```python
from build123d import *

# Parameters (mm, degrees)
SKETCH1_W           = 24
SKETCH1_H           = 24
BOSS_EXTRUDE1_DEPTH = 20
SKETCH5_W           = 5
SKETCH5_H           = 4
SKETCH3_W           = 20
SKETCH3_H           = 20
CUT_EXTRUDE5_DEPTH  = 6
SKETCH14_W          = 20
SKETCH14_H          = 20
CUT_EXTRUDE6_DEPTH  = 2
CUT_EXTRUDE7_REACH  = 14
SKETCH15_W          = 17.5
SKETCH15_H          = 17.5


with BuildPart() as part:
    # Sketch1 → Boss-Extrude1 (new body)
    with BuildSketch(Plane(origin=(0, 0, 0), x_dir=(1, 0, 0), z_dir=(0, 1, 0))):
        Rectangle(SKETCH1_W, SKETCH1_H)
    extrude(amount=BOSS_EXTRUDE1_DEPTH)

    # Sweep1: sweep along a path in Sketch6
    with BuildLine(Plane(origin=(0, 0, 0), x_dir=(0, 0, -1), z_dir=(1, 0, 0))) as sweep1_path:
        Line((12, 16), (15, 16))
        ThreePointArc((15, 16), (17.025627927, 16.352272006), (18.813398517, 17.367722833))
    # Sketch5 → Sweep1 (sweep)
    with BuildSketch(Plane(origin=(0, 0, -12), x_dir=(-1, 0, 0), z_dir=(0, 0, -1))):
        with Locations((0, 16)):
            Rectangle(SKETCH5_W, SKETCH5_H)
    sweep1 = sweep(path=sweep1_path.line)

    # Mirror1: Sweep1 across plane
    add(sweep1.mirror(Plane.XY))

    # Sketch3 → Cut-Extrude5 (cut)
    with BuildSketch(Plane.XZ):
        Rectangle(SKETCH3_W, SKETCH3_H)
    extrude(amount=-CUT_EXTRUDE5_DEPTH, mode=Mode.SUBTRACT)

    # Sketch14 → Cut-Extrude6 (cut)
    with BuildSketch(Plane.XZ.offset(-6)):
        Rectangle(SKETCH14_W, SKETCH14_H)
    extrude(amount=-CUT_EXTRUDE6_DEPTH, mode=Mode.SUBTRACT)

    # Sketch15 → Cut-Extrude7 (cut, up to next)
    with BuildSketch(Plane.XZ.offset(-8), mode=Mode.PRIVATE) as cut_extrude7_sk1:
        Rectangle(SKETCH15_W, SKETCH15_H)
    cut_extrude7_tool1 = extrude(cut_extrude7_sk1.sketch, amount=-CUT_EXTRUDE7_REACH, mode=Mode.PRIVATE) & part.part
    add(cut_extrude7_tool1.solids().sort_by_distance((0, 8, 0))[0], mode=Mode.SUBTRACT)


solid = part.part
```
For this review, take the finished solid that the model builds, in its own axes (mm). A direction names the side the tool comes from. Give positions to 0.01 mm unless a question says otherwise; leave off trailing zeros. Order: outer loops, then holes, each group sorted by start corner. A loop starts at its lowest first (then second) coordinate and runs counter-clockwise, first axis right, second up.
1) The part is to be moulded in two halves that separate along Z. For faces 1 (the face through (-9, 8, 0)), 2 (the face through (-0.035, 14.457, 17.665)), 3 (the face through (0, 14, -8.75)), 4 (the face through (-0.035, 17.389, -18.796)), say which applies: released by +Z, released by -Z, zero draft, split by the parting line, or undercut.
2) Insertion check: pin 1 (4 mm diameter, centred on x = 1.5, y = 3, fed in from -Z); pin 2 (2 mm diameter, centred on x = 4, y = 11.5, fed in from +Z); pin 3 (1.5 mm diameter, centred on y = 17, z = -17.5, fed in from -X). Each pin has a flat end and moves straight along its axis. Give the tip position at first contact, or say it passes through.
3) Take a section at A-A (x = 6.75). Give the boundary of the cut face in (y, z).
4) Take a section at C-C (y = 10). Give the boundary of the cut face in (x, z).
5) Take a section at D-D (x = -9.5). Give the boundary of the cut face in (y, z).
6) For faces 5 (the face through (-2.5, 16, -15)), 6 (the face through (-8.75, 14, 0)), 7 (the face through (0, 14, -14)), 8 (the face through (0, 4, 10)), list the 3-axis set-ups (+Z, -Z, +X, -X, +Y, -Y) from which the entire face can be reached by the end or side of a thin tool; tool diameter is ignored.
7) Wall thickness on line 1 (Z direction, x = 4, y = 16.25); line 2 (X direction, y = 5.25, z = 2.5): over which ranges is each line inside the solid? List them lowest first.
8) Take a section at B-B (z = -7). Give the boundary of the cut face in (x, y).
Derived:
1. face 1: undercut
1. face 2: released by +Z
1. face 3: undercut
1. face 4: released by -Z
2. pin 1: stops at z = -12
2. pin 2: stops at z = 12
2. pin 3: stops at x = -2.5
3. outline: (0, -12) - (20, -12) - (20, -8.75) - (8, -8.75) - (8, -10) - (0, -10) - close; (0, 10) - (8, 10) - (8, 8.75) - (20, 8.75) - (20, 12) - (0, 12) - close
4. outline: (-12, -12) - (12, -12) - (12, 12) - (-12, 12) - close; hole (-8.75, -8.75) - (8.75, -8.75) - (8.75, 8.75) - (-8.75, 8.75) - close
5. outline: (0, -12) - (20, -12) - (20, 12) - (0, 12) - (0, 10) - (8, 10) - (8, -10) - (0, -10) - close
6. face 5: -Z, -X, +Y, -Y
6. face 6: +Y, -Y
6. face 7: -Z, +X, -X, -Y
6. face 8: -Y
7. line 1: z = -12 to -8.75, 8.75 to 12
7. line 2: x = -12 to -10, 10 to 12
8. outline: (-12, 0) - (-10, 0) - (-10, 8) - (-8.75, 8) - (-8.75, 20) - (-12, 20) - close; (8.75, 8) - (10, 8) - (10, 0) - (12, 0) - (12, 20) - (8.75, 20) - close
